from build123d import *

# Parameters (mm, degrees)
F1_DEPTH = 12.7
F2_R     = 6.35
F3_DEPTH = 12.7


with BuildPart() as f1:
    # F0 (on Top) → F1 (new body)
    with BuildSketch(Plane.XY):
        with BuildLine():
            ThreePointArc((21.997045, 12.7), (12.7, 21.997045), (0, 25.4))
            ThreePointArc((0, 25.4), (-25.4, 0), (0, -25.4))
            ThreePointArc((0, -25.4), (8.412257, -23.966517), (15.875, -19.827869))
            Line((15.875, -19.827869), (15.875, -12.7))
            Line((15.875, -12.7), (0, -12.7))
            ThreePointArc((0, -12.7), (-12.7, 0), (0, 12.7))
            Line((0, 12.7), (21.997045, 12.7))
        make_face()
        with BuildLine():
            Line((63.5, 25.4), (0, 25.4))
            ThreePointArc((0, 25.4), (12.7, 21.997045), (21.997045, 12.7))
            Line((21.997045, 12.7), (41.502955, 12.7))
            ThreePointArc((41.502955, 12.7), (50.8, 21.997045), (63.5, 25.4))
        make_face()
        with BuildLine():
            ThreePointArc((88.9, 0), (81.460512, 17.960512), (63.5, 25.4))
            ThreePointArc((63.5, 25.4), (50.8, 21.997045), (41.502955, 12.7))
            Line((41.502955, 12.7), (63.5, 12.7))
            ThreePointArc((63.5, 12.7), (72.480256, 8.980256), (76.2, 0))
            ThreePointArc((76.2, 0), (72.480256, -8.980256), (63.5, -12.7))
            Line((63.5, -12.7), (63.5, -25.4))
            ThreePointArc((63.5, -25.4), (81.460512, -17.960512), (88.9, 0))
        make_face()
        with BuildLine():
            ThreePointArc((63.5, -25.4), (55.087743, -23.966517), (47.625, -19.827869))
            Line((47.625, -19.827869), (47.625, -25.4))
            Line((47.625, -25.4), (63.5, -25.4))
        make_face()
        with BuildLine():
            ThreePointArc((15.875, -19.827869), (8.412257, -23.966517), (0, -25.4))
            Line((0, -25.4), (15.875, -25.4))
            Line((15.875, -25.4), (15.875, -19.827869))
        make_face()
        with BuildLine():
            Line((47.625, -12.7), (47.625, -19.827869))
            ThreePointArc((47.625, -19.827869), (55.087743, -23.966517), (63.5, -25.4))
            Line((63.5, -25.4), (63.5, -12.7))
            Line((63.5, -12.7), (47.625, -12.7))
        make_face()
    extrude(amount=F1_DEPTH)

    # F2 (on face) → F3 (join, through all)
    with BuildSketch(Plane(origin=(0, 25.4, 0), x_dir=(-1, 0, 0), z_dir=(0, 1, 0))):
        with BuildLine():
            ThreePointArc((-47.625, -12.7), (-31.75, -28.575), (-15.875, -12.7))
            ThreePointArc((-15.875, -12.7), (-31.75, 3.175), (-47.625, -12.7))
        make_face()
        with Locations((-31.75, -12.7)):
            Circle(F2_R, mode=Mode.SUBTRACT)
        with BuildLine():
            ThreePointArc((-22.225, 0), (-17.550968, -5.600484), (-15.875, -12.7))
            Line((-15.875, -12.7), (-15.875, 0))
            Line((-15.875, 0), (-22.225, 0))
        make_face()
        with BuildLine():
            Line((-47.625, 0), (-47.625, -12.7))
            ThreePointArc((-47.625, -12.7), (-45.949032, -5.600484), (-41.275, 0))
            Line((-41.275, 0), (-47.625, 0))
        make_face()
    extrude(amount=-F3_DEPTH)


solid = f1.part
The model under review builds one solid part; all positions refer to its coordinate system, in mm. A direction names the side the tool comes from. Give positions to 0.01 mm unless a question says otherwise; leave off trailing zeros. Loops run counter-clockwise (first coordinate to the right, second up) from the corner with the lowest first, then second, coordinate; pieces in that order, holes last. Notation, with made-up numbers: (9.25, 28.5) -> (54.25, 28.5) arc R24 cw to (54.25, 53.5) -> close; hole circle Ø8 at (60, 84.25). An arc over 180 degrees is marked (long way). Answer as a JSON object with one key per item and string values. Group by question number.
Q1. Take a section at B-B (z = -9). Write out the cut boundary in (x, y) (3 decimals), plus the area to 3 significant figures.
Q2. Tool access review of faces 4 (the flat face through (-14, 0, 0)), 5 (the flat face through (15.875, -19, 6)), 6 (the flat face through (8, -12.7, 6)), 7 (the flat face through (47.625, 19, -6)): name each direction out of +Z, -Z, +X, -X, +Y, -Y from which nothing blocks a thin tool from reaching the whole face with its end or side.
Q3. Take a section at C-C (y = 19). Write out the cut boundary in (x, z) (3 decimals).
Q4. Take a section at D-D (x = -16). Write out the cut boundary in (y, z).
Q5. Draft analysis for pull direction Y (two halves, no side actions). For faces 1 (the cylindrical face through (-25.394, 0.559, 6.261)), 2 (the flat face through (31, 17, 12.7)), 3 (the flat face through (32, 12.7, -3)), state which applies: pulls with the +Y half, pulls with the -Y half, needs draft (parallel to the pull), parting line crosses it, or undercut.
Q6. Wall thickness on line 1 along Z through (x, y) = (31.75, 18.5) (3 decimals); line 2 along Z through (x, y) = (-15, -17.5); line 3 along X through (y, z) = (-2.5, 6.5): over which ranges is each line inside the solid? List them lowest first.
Q7. Insertion check: pin 1 (4 mm diameter, centred on y = -20, z = 6, fed in from -X); pin 2 (1 mm diameter, centred on x = 76.5, y = 2, fed in from -Z); pin 3 (1 mm diameter, centred on x = 66.5, y = -11, fed in from -Z); pin 4 (14 mm diameter, centred on y = -21, z = 6, fed in from +X). Each pin has a flat end and moves straight along its axis. Give the tip position at first contact, or say it passes through.
Q8. Take a section at A-A (x = 50). Write out the cut boundary in (y, z), plus the area to 3 significant figures.
Answer below:
{
 "1": {"outline": "(15.875, 12.7) -> (26.589, 12.7) -> (26.589, 25.4) -> (15.875, 25.4) -> close; (36.911, 12.7) -> (47.625, 12.7) -> (47.625, 25.4) -> (36.911, 25.4) -> close", "area": "272 mm2"},
 "2": {"face 4": "-Z, -X, +Y, -Y", "face 5": "+Z, -Z, -Y", "face 6": "+Z, -Z", "face 7": "-Z, +X, +Y, -Y"},
 "3": {"outline": "(-16.857, 0) -> (15.875, 0) -> (15.875, -12.7) arc R15.875 ccw to (47.625, -12.7) -> (47.625, 0) -> (80.357, 0) -> (80.357, 12.7) -> (-16.857, 12.7) -> close; hole circle Ø12.7 at (31.75, -12.7)"},
 "4": {"outline": "(-19.73, 0) -> (19.73, 0) -> (19.73, 12.7) -> (-19.73, 12.7) -> close"},
 "5": {"face 1": "parting line crosses it", "face 2": "needs draft", "face 3": "undercut"},
 "6": {"line 1": "z = -28.575 to -19.05, -6.35 to 12.7", "line 2": "z = 0 to 12.7", "line 3": "x = -25.28 to -12.45, 75.95 to 88.78"},
 "7": {"pin 1": "stops at x = -17.92", "pin 2": "stops at z = 0", "pin 3": "passes through", "pin 4": "stops at x = 84.69"},
 "8": {"outline": "(-25.4, 0) -> (-12.7, 0) -> (-12.7, 12.7) -> (-25.4, 12.7) -> close; (12.7, 0) -> (25.4, 0) -> (25.4, 12.7) -> (12.7, 12.7) -> close", "area": "323 mm2"}
}
